Design review of the part shown in the three views and the two pictorial views. Dimensions are in mm from the part's minimum x, y and z. Coordinates: 2 decimals unless noted, no trailing zeros. Loops run counter-clockwise (first coordinate to the right, second up) from the corner with the lowest first, then second, coordinate; pieces in that order, holes last. Notation, with made-up numbers: (-37.5, 3) - (-27.5, 3) arc R19 ccw to (-27.5, 33) - close; hole circle Ø3 at (74.5, -24). An arc over 180 degrees is marked (long way). One line per item, written item: value. Start each with the question number.
1. Take a section at A-A, the plane y = 105.5. State the section outline as (x, z) points (1 decimal), and give its area (3 significant figures).
2. To check wall thickness, follow line 1 (Y direction, x = 82, z = 1.95) (1 decimal); line 2 (X direction, y = 79, z = 0.25) (1 decimal); line 3 (Y direction, x = 26, z = 0.65) (1 decimal). State the ranges of each line that lie inside material, in increasing order. Write a range as from..to.
3. Insertion check: pin 1 (1 mm diameter, centred on y = 125.5, z = 0.5, fed in from +X); pin 2 (1 mm diameter, centred on y = 48.5, z = 1, fed in from +X). Each pin has a flat end and moves straight along its axis. Give the tip position at first contact, or say it passes through.
4. Take a section at B-B, the plane x = 128. State the section outline as (y, z) points.
5. Take a section at C-C, the plane z = 1.6. Count the separate pieces of the cut face and the enclosed holes in it, and give its area (3 significant figures).
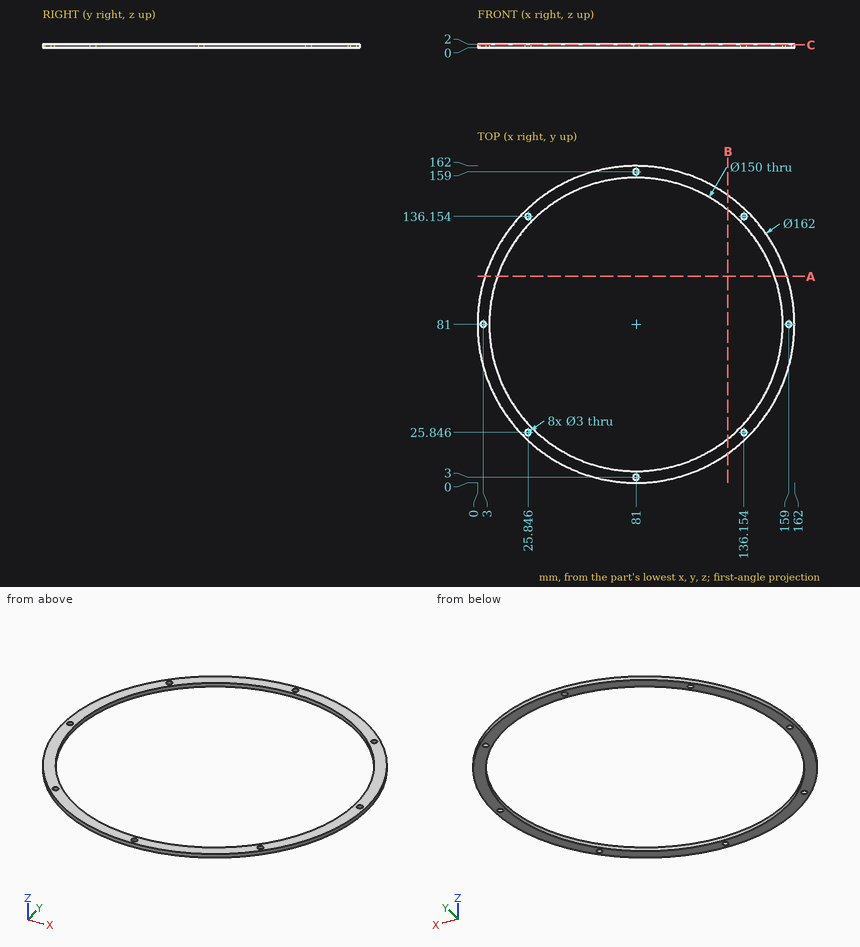
Solutions:
1. outline: (3.8, 0) - (10.1, 0) - (10.1, 2) - (3.8, 2) - close; (151.9, 0) - (158.2, 0) - (158.2, 2) - (151.9, 2) - close
1. area: 25.3 mm2
2. line 1: 0..1.9, 4.1..6, 156..157.9, 160.1..162
2. line 2: 0..6, 156..162
2. line 3: 21.5..24.4, 27.3..30, 132..134.7, 137.6..140.5
3. pin 1: x = 149.01
3. pin 2: x = 155.41
4. outline: (15.03, 0) - (22.55, 0) - (22.55, 2) - (15.03, 2) - close; (139.45, 0) - (146.97, 0) - (146.97, 2) - (139.45, 2) - close
5. separate pieces: 1
5. enclosed holes: 9
5. area: 2,880 mm2
